from build123d import *

# Parameters (mm, degrees)
EXTRUDE_1_DEPTH = 4.2
FILLET_1_R      = 1.8
SHELL_1_T       = -1


with BuildPart() as part:
    # 草图1 → 凸台-拉伸1 (new body)
    with BuildSketch(Plane(origin=(0, 0, 0), x_dir=(1, 0, 0), z_dir=(0, 1, 0))):
        with BuildLine():
            Line((-30.7, 16.15), (30.7, 16.15))
            ThreePointArc((30.7, 16.15), (32.255634919, 15.505634919), (32.9, 13.95))
            Line((32.9, 13.95), (32.9, -13.95))
            ThreePointArc((32.9, -13.95), (32.255634919, -15.505634919), (30.7, -16.15))
            Line((30.7, -16.15), (-30.7, -16.15))
            ThreePointArc((-30.7, -16.15), (-32.255634919, -15.505634919), (-32.9, -13.95))
            Line((-32.9, -13.95), (-32.9, 13.95))
            ThreePointArc((-32.9, 13.95), (-32.255634919, 15.505634919), (-30.7, 16.15))
        make_face()
    extrude(amount=EXTRUDE_1_DEPTH)

    # 圆角1
    fillet_1_edges = [part.edges().sort_by_distance(p)[0] for p in [
        (32.255634919, 4.2, 15.505634919),
        (32.9, 4.2, 0),
        (32.255634919, 4.2, -15.505634919),
        (0, 4.2, -16.15),
        (-32.255634919, 4.2, -15.505634919),
        (-32.9, 4.2, 0),
        (-32.255634919, 4.2, 15.505634919),
        (0, 4.2, 16.15),
    ]]
    fillet(fillet_1_edges, radius=FILLET_1_R)

    # 抽壳1
    shell_1_openings = [part.faces().sort_by_distance(p)[0] for p in [
        (0, 0, 0),
    ]]
    offset(amount=SHELL_1_T, openings=shell_1_openings, kind=Kind.INTERSECTION)


solid = part.part
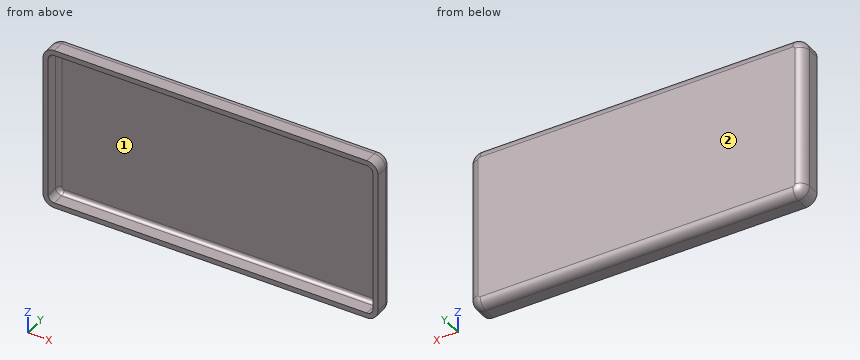
Verification items for the finished model (mm, model axes). Face numbers are marked on the shaded views. Coordinates: 2 decimals unless noted, no trailing zeros. Order: outer loops, then holes, each group sorted by start corner. A loop starts at its lowest first (then second) coordinate and runs counter-clockwise, first axis right, second up. Notation, with made-up numbers: (72, -28.75) -> (112, -28.75) arc R10 cw to (112, -24.75) -> close; hole circle Ø2 at (-27.75, 22). An arc over 180 degrees is marked (long way). Use CSV: the item, a comma, the result in double quotes. Start each with the question number.
Q1. Draft check along X on the marked faces 1 and 2. Enter one of: +X half, -X half, draft (parallel to the pull), parting line (faces both ways), or undercut.
Q2. Thickness scan on line 1 along X through (y, z) = (0.5, -9); line 2 along Z through (x, y) = (3, 2.3); line 3 along Y through (x, z) = (-8.5, 6.5). Record the ranges inside material, lowest first.
Q3. Section check C-C, the plane y = 1.1. Record the cut outline in (x, z), and give its area (3 significant figures).
Q4. Section check B-B, the plane z = -2.5. Record the cut outline in (x, y), and give its area (3 significant figures).
Q5. Section check A-A, the plane x = -17. Record the cut outline in (y, z), and give its area (3 significant figures).
Q6. Depth check by flat-ended pin: P1, Ø10, axis at x = -5.5, z = -9, coming from the -Y side; P2, Ø1, axis at x = 23.5, y = 3.5, coming from the -Z side. Enter the tip coordinate at first touch or a pass-through.
Returned:
1,face 1,"undercut"
1,face 2,"draft"
2,line 1,"x = -32.9 to -31.9, 31.9 to 32.9"
2,line 2,"z = -16.15 to -15.15, 15.15 to 16.15"
2,line 3,"y = 3.2 to 4.2"
3,outline,"(-32.9, -13.95) arc R2.2 ccw to (-30.7, -16.15) -> (30.7, -16.15) arc R2.2 ccw to (32.9, -13.95) -> (32.9, 13.95) arc R2.2 ccw to (30.7, 16.15) -> (-30.7, 16.15) arc R2.2 ccw to (-32.9, 13.95) -> close; hole (-31.9, -13.95) arc R1.2 ccw to (-30.7, -15.15) -> (30.7, -15.15) arc R1.2 ccw to (31.9, -13.95) -> (31.9, 13.95) arc R1.2 ccw to (30.7, 15.15) -> (-30.7, 15.15) arc R1.2 ccw to (-31.9, 13.95) -> close"
3,area,"189 mm^2"
4,outline,"(-32.9, 0) -> (-31.9, 0) -> (-31.9, 2.4) arc R0.8 cw to (-31.1, 3.2) -> (31.1, 3.2) arc R0.8 cw to (31.9, 2.4) -> (31.9, 0) -> (32.9, 0) -> (32.9, 2.4) arc R1.8 ccw to (31.1, 4.2) -> (-31.1, 4.2) arc R1.8 ccw to (-32.9, 2.4) -> close"
4,area,"71.1 mm^2"
5,outline,"(0, -16.15) -> (2.4, -16.15) arc R1.8 ccw to (4.2, -14.35) -> (4.2, 14.35) arc R1.8 ccw to (2.4, 16.15) -> (0, 16.15) -> (0, 15.15) -> (2.4, 15.15) arc R0.8 cw to (3.2, 14.35) -> (3.2, -14.35) arc R0.8 cw to (2.4, -15.15) -> (0, -15.15) -> close"
5,area,"37.6 mm^2"
6,P1,"stops at y = 3.2"
6,P2,"stops at z = -16.05"
